from build123d import *

# Parameters (mm, degrees)
F1_DEPTH = 5.55625
F3_R     = 1.27
F4_DEPTH = 3.175
F5_R     = 1.27
F6_DEPTH = 2.38125
F2_R     = 1.27
F7_DEPTH = 2.778125


with BuildPart() as f1:
    # F0 (on Top) → F1 (new body)
    with BuildSketch(Plane.XY):
        with BuildLine():
            Line((-5.55625, 0), (-1.0033, 0))
            ThreePointArc((-1.0033, 0), (-0.70944, 0.70944), (0, 1.0033))
            Line((0, 1.0033), (0, 5.55625))
            Line((0, 5.55625), (-5.55625, 5.55625))
            Line((-5.55625, 5.55625), (-5.55625, 0))
        make_face()
    extrude(amount=F1_DEPTH)

    # F3 (on face) → F4 (cut)
    with BuildSketch(Plane.XZ):
        with Locations((-3.279775, 3.7338)):
            Circle(F3_R)
    extrude(amount=-F4_DEPTH, mode=Mode.SUBTRACT)

    # F5 (on face) → F6 (cut)
    with BuildSketch(Plane(origin=(0, 0, 0), x_dir=(1, 0, 0), z_dir=(0, 0, -1))):
        with Locations((-3.279775, -3.279775)):
            Circle(F5_R)
    extrude(amount=-F6_DEPTH, mode=Mode.SUBTRACT)

    # F2 (on face) → F7 (join)
    with BuildSketch(Plane.YZ):
        with Locations((3.279775, 3.7338)):
            Circle(F2_R)
    extrude(amount=F7_DEPTH)


with BuildPart() as f8_1:
    # F8: copy of F1
    add(f1.part.moved(Location((25.4, 0, 0))))


solid = f1.part
Work out the finished part from the listing and answer in its coordinate system (mm). A direction names the side the tool comes from. Give positions to 0.01 mm unless a question says otherwise; leave off trailing zeros. Loops run counter-clockwise (first coordinate to the right, second up) from the corner with the lowest first, then second, coordinate; pieces in that order, holes last. Notation, with made-up numbers: (-13.5, 50) -> (-5.5, 50) arc R26 cw to (-5.5, 84) -> close; hole circle Ø9 at (-6.5, 83). An arc over 180 degrees is marked (long way). Use a Markdown table: item, result. Add a question column.
1. Section A-A on y = 2.65 is taken. Determine the outline of the cut face in (x, z).
2. Section C-C on x = -3.5 is taken. Determine the outline of the cut face in (y, z) (3 decimals), and give its area (3 significant figures).
3. Determine the mould class of faces 4 (the flat face through (-3, 5.556, 3)), 5 (the flat face through (-3.3, 3.3, 2.381)), 6 (the flat face through (-5.556, 3, 3)) for opening direction Y: released by +Y, released by -Y, zero draft, split by the parting line, or undercut.
4. Section B-B on z = 0.45 is taken. Determine the outline of the cut face in (x, y).
5. A flat-ended cylindrical pin translates along its axis: pin 1 Ø0.8 at (x, z) = (-3.5, 3.5) entering from -Y (3 decimals). Find the tip coordinate at first contact, or state that the pin passes through.
6. Section D-D on z = 2.75 is taken. Determine the outline of the cut face in (x, y) (3 decimals), and give its area (3 significant figures).
7. Find the intervals of material crossed by probe 1 along Y at (x, z) = (-3.25, 1.7); probe 2 along X at (y, z) = (1.4, 3.75); probe 3 along Y at (x, z) = (-3, 2.7) (3 decimals), in increasing order.
8. For faces 1 (the cylindrical face through (-3.555, 1.565, 2.494)), 2 (the cylindrical face through (1.37, 3.87, 2.61)), 3 (the cylindrical face through (-3.45, 2.02, 1.17)), determine the directions among +Z, -Z, +X, -X, +Y, -Y from which every point of the face is accessible in a straight line to the end or side of a thin tool.
Results below:
| question | item | result |
|---|---|---|
| 1 | outline | (-5.56, 0) -> (-4.38, 0) -> (-4.38, 2.38) -> (-2.18, 2.38) -> (-2.18, 0) -> (0, 0) -> (0, 2.63) -> (2.78, 2.63) -> (2.78, 4.84) -> (0, 4.84) -> (0, 5.56) -> (-5.56, 5.56) -> close; hole circle Ø2.54 at (-3.28, 3.73) |
| 2 | outline | (0, 0) -> (2.029, 0) -> (2.029, 2.381) -> (4.531, 2.381) -> (4.531, 0) -> (5.556, 0) -> (5.556, 5.556) -> (0, 5.556) -> (0, 4.985) -> (3.175, 4.985) -> (3.175, 2.483) -> (0, 2.483) -> close |
| 2 | area | 17.0 mm^2 |
| 3 | face 4 | released by +Y |
| 3 | face 5 | undercut |
| 3 | face 6 | zero draft |
| 4 | outline | (-5.56, 0) -> (-1, 0) arc R1 cw to (0, 1) -> (0, 5.56) -> (-5.56, 5.56) -> close; hole circle Ø2.54 at (-3.28, 3.28) |
| 5 | pin 1 | stops at y = 3.175 |
| 6 | outline | (-5.556, 0) -> (-4.083, 0) -> (-4.083, 3.175) -> (-2.477, 3.175) -> (-2.477, 0) -> (-1.003, 0) arc R1.003 cw to (0, 1.003) -> (0, 2.477) -> (2.778, 2.477) -> (2.778, 4.083) -> (0, 4.083) -> (0, 5.556) -> (-5.556, 5.556) -> close |
| 6 | area | 29.4 mm^2 |
| 7 | probe 1 | y = 0 to 2.01, 4.55 to 5.56 |
| 7 | probe 2 | x = -5.56 to -4.55, -2.01 to 0 |
| 7 | probe 3 | y = 3.175 to 5.556 |
| 8 | face 1 | -Y |
| 8 | face 2 | +X |
| 8 | face 3 | -Z |
